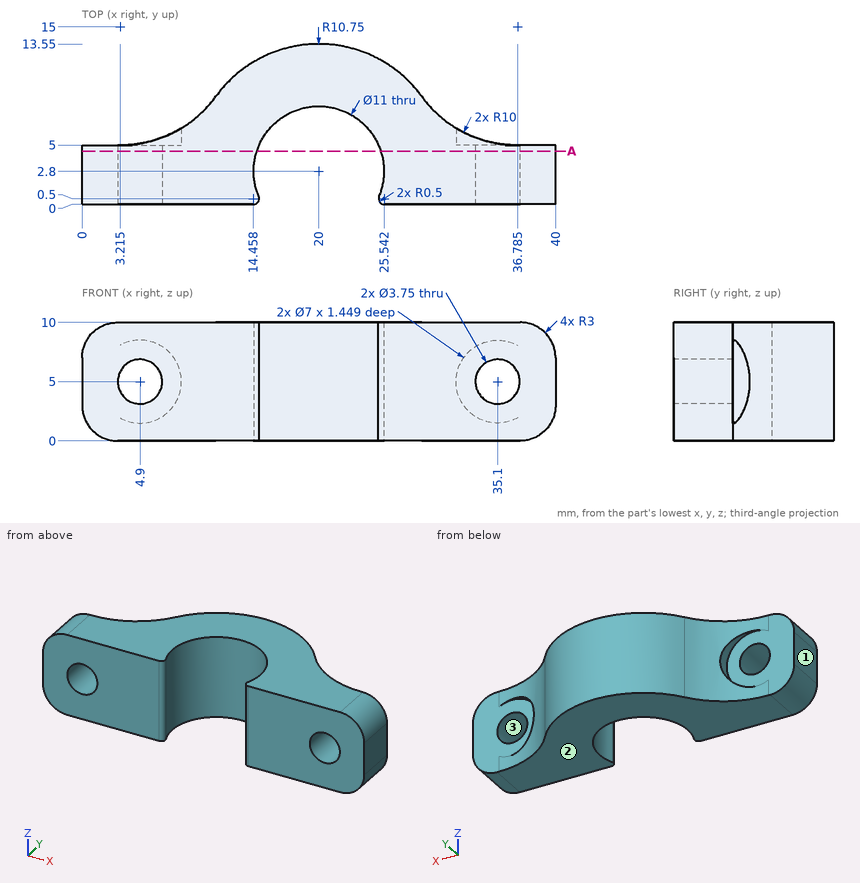
Geometry: see drawing. Coordinates: mm, zero at the bounding-box minimum. Coordinates: 2 decimals unless noted, no trailing zeros. Answer in a Markdown table with one row per item.
(1) Mould query, pull axis Z, two halves, no side actions, for the marked faces 1, 2 and 3. Classes: pulls with the +Z half, pulls with the -Z half, needs draft (parallel to the pull), parting line crosses it, or undercut.
Model answer:
| item | result |
|---|---|
| face 1 | needs draft |
| face 2 | pulls with the -Z half |
| face 3 | undercut |
(2) Pin query (flat end, axial travel): P1, Ø3, axis at y = 6, z = 9, coming from the +X side; P2, Ø1.5, axis at y = 7, z = 9, coming from the -X side (1 decimal); P3, Ø6, axis at x = 35.1, z = 5, coming from the +Y side; P4, Ø2, axis at x = 4.9, z = 5, coming from the +Y side. Return the tip coordinate at first contact, or that it passes through.
Model answer:
| item | result |
|---|---|
| P1 | stops at x = 39.87 |
| P2 | stops at x = 8.1 |
| P3 | stops at y = 5 |
| P4 | passes through |
(3) Cut plane A-A on y = 4.5. Count the separate pieces of the cut face and the enclosed holes in it.
Model answer:
| item | result |
|---|---|
| separate pieces | 2 |
| enclosed holes | 2 |
(4) Material intervals for L1, parallel to X at y = 2.95, z = 5 (1 decimal); L2, parallel to Z at x = 5, y = 1; L3, parallel to X at y = 2.5, z = 4.25, sorted ascending. Write a range as from..to.
Model answer:
| item | result |
|---|---|
| L1 | x = 0..3, 6.8..14.5, 25.5..33.2, 37..40 |
| L2 | z = 0..3.13, 6.87..10 |
| L3 | x = 0..3.18, 6.62..14.51, 25.49..33.38, 36.82..40 |
